Model file for the job. Use its own axes, mm. A direction names the side the tool comes from. Round coordinates to 2 decimals unless told otherwise and drop trailing zeros. Order: outer loops, then holes, each group sorted by start corner. A loop starts at its lowest first (then second) coordinate and runs counter-clockwise, first axis right, second up. Notation, with made-up numbers: (47.25, 87.25) -> (59.25, 87.25) arc R27 ccw to (59.25, 125.25) -> close; hole circle Ø5 at (-22, 20). An arc over 180 degrees is marked (long way). Put each result on its own line as item: value. Start each with the question number.
Q1. Cut at A-A, the plane x = 0. List the corners of the cut face in (y, z).
Q2. Flat gauge pins, fed straight in: P1, Ø8, axis at y = -23, z = 7.5, coming from the -X side; P2, Ø2, axis at x = 0.5, z = 41.5, coming from the +Y side; P3, Ø5, axis at y = 0, z = 22.5, coming from the -X side. Where does each tip first touch, or does it go through?
Q3. Cut at B-B, the plane y = -20. State how many separate pieces and enclosed holes the cut face has, and give its area (3 significant figures).
Q4. Pull direction Z, two halves, no side cores. Call faces 3 (the face through (0, -48, 0)), 4 (the face through (-0.54, -20.43, 21.92)): released by +Z, released by -Z, zero draft, split by the parting line, or undercut.
Q5. Probe L1, parallel to Z at x = -1.5, y = -8; L2, parallel to Y at x = -1, z = 5.5; L3, parallel to Z at x = 1, y = 11. List the from-to ranges inside material, lowest first.
Q6. 3-axis set-ups, long thin cutter, end or side, ignore diameter. For faces 1 (the face through (-0.54, 19.57, 21.92)), 2 (the face through (0, 0, 0)): which of +Z, -Z, +X, -X, +Y, -Y reach the whole face in a straight line?
from build123d import *

# Parameters (mm, degrees)
F1_R     = 3.5
F3_R     = 3
F4_DEPTH = 46
F5_R     = 2.5
F6_DEPTH = 40.5
F7_R     = 2.5
F8_DEPTH = 45


with BuildPart() as f2:
    # F2: sweep along a path in F0
    with BuildLine(Plane.YZ) as f2_path:
        ThreePointArc((44.654696, 0), (-0.345304, 45), (-45.345304, 0))
    # F1 (on Top) → F2 (sweep)
    with BuildSketch(Plane.XY):
        with Locations((0, -47.845304)):
            Circle(F1_R)
    sweep(path=f2_path.line)

    # F3 (on Top) → F4 (join)
    with BuildSketch(Plane.XY):
        Circle(F3_R)
    extrude(amount=F4_DEPTH)

    # F5 (on Front) → F6 (join, symmetric)
    with BuildSketch(Plane.XZ):
        with Locations((0, 24.36039)):
            Circle(F5_R)
    extrude(amount=F6_DEPTH, both=True)

    # F7 (on Front) → F8 (join, symmetric)
    with BuildSketch(Plane.XZ):
        with Locations((0, 8)):
            Circle(F7_R)
    extrude(amount=F8_DEPTH, both=True)


solid = f2.part
Ans:
1. outline: (-51.35, 0) -> (-44.35, 0) arc R44 cw to (-44, 5.5) -> (-3, 5.5) -> (-3, 0) -> (3, 0) -> (3, 5.5) -> (43.31, 5.5) arc R44 cw to (43.65, 0) -> (50.65, 0) arc R51 ccw to start; hole (-43.07, 10.5) -> (-3, 10.5) -> (-3, 21.86) -> (-38.53, 21.86) arc R44 ccw to start; hole (-35.2, 26.86) -> (-3, 26.86) -> (-3, 43.92) arc R44 ccw to start; hole (3, 10.5) -> (42.38, 10.5) arc R44 ccw to (37.84, 21.86) -> (3, 21.86) -> close; hole (3, 26.86) -> (34.5, 26.86) arc R44 ccw to (3, 43.87) -> close
2. P1: stops at x = -2.5
2. P2: stops at y = 30.61
2. P3: stops at x = -3
3. separate pieces: 3
3. enclosed holes: 0
3. area: 81.6 mm^2
4. face 3: released by -Z
4. face 4: undercut
5. L1: z = 6 to 10, 22.36 to 26.36, 43.67 to 50.08
5. L2: y = -50.9 to -44.15, -2.83 to 2.83, 43.46 to 50.21
5. L3: z = 5.71 to 10.29, 22.07 to 26.65, 42.66 to 49.57
6. face 1: none
6. face 2: -Z, +X, -X, +Y, -Y
